from build123d import *

# Parameters (mm, degrees)
FILLET2_R  = 0.1
SKETCH2_W  = 5.5
SKETCH2_H  = 0.8
SLOT_DEPTH = 0.85


with BuildPart() as part:
    # BodySke → Base-Revolve (revolve)
    with BuildSketch(Plane.XY):
        Polygon((2, 1.5), (2, 2.75), (0, 2.575022673), (0, 0), (18, 0), (18, 1.5), align=None)
    revolve(axis=Axis((-25.4, 0, 0), (1, 0, 0)))

    # Fillet2
    fillet2_edges = [part.edges().sort_by_distance(p)[0] for p in [
        (0, -2.575022673, 0),
    ]]
    fillet(fillet2_edges, radius=FILLET2_R)

    # Sketch2 → Slot (cut)
    with BuildSketch(Plane(origin=(0, 0, 0), x_dir=(0, 0, -1), z_dir=(1, 0, 0))):
        Rectangle(SKETCH2_W, SKETCH2_H)
    extrude(amount=SLOT_DEPTH, mode=Mode.SUBTRACT)


solid = part.part
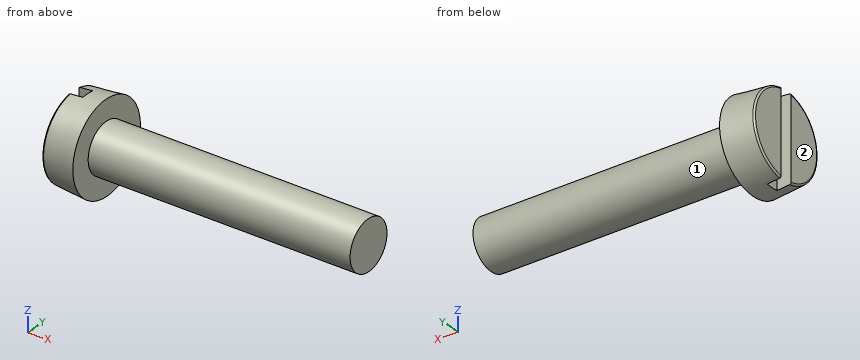
Source: CAD feature listing. Evaluate the final solid. Frame: model axes, mm. Face numbers are marked on the shaded views. A direction names the side the tool comes from. Give positions to 0.01 mm unless a question says otherwise; leave off trailing zeros. Write each loop counter-clockwise with the first axis right and the second up, starting at its lowest first coordinate (ties: lowest second). Pieces come first, ordered by that corner, then holes. Notation, with made-up numbers: M 11.25,42 L 40.25,42 A16 ccw 40.25,58 Z; hole C 50,-10 d1. An arc over 180 degrees is marked long. Return JSON: item names as keys, results as strings. Group by question number.
1) Cut plane A-A, the plane z = 0. Output: boundary loops of the cut face in (x, y).
2) Ray query, L1, parallel to X at y = -1.25, z = 1.5; L2, parallel to Y at x = 4.5, z = 0.1; L3, parallel to Z at x = 2.5, y = -0.8. Return the intervals inside material, ascending.
3) Cut plane C-C, the plane x = 16. Output: boundary loops of the cut face in (y, z).
4) Set-up query: the marked faces 1 and 2. Return all of +Z, -Z, +X, -X, +Y, -Y with unobstructed straight access to the full face (end or side cutting, diameter ignored); none if empty.
5) First-contact query: pin 1 Ø2 at (x, y) = (12, -1) entering from +Z; pin 2 Ø1.5 at (x, y) = (4.5, -1.5) entering from +Z. Flat tips, straight axial feed; report the tip coordinate or a pass-through.
6) Cut plane B-B, the plane y = 0. Output: boundary loops of the cut face in (x, z).
Data:
{
 "1": {"outline": "M 0,-2.48 A0.1 ccw 0.09,-2.58 L 2,-2.75 L 2,-1.5 L 18,-1.5 L 18,1.5 L 2,1.5 L 2,2.75 L 0.09,2.58 A0.1 ccw 0,2.48 L 0,0.4 L 0.85,0.4 L 0.85,-0.4 L 0,-0.4 Z"},
 "2": {"L1": "x = 0 to 2", "L2": "y = -1.5 to 1.5", "L3": "z = -1.27 to 1.27"},
 "3": {"outline": "C 0,0 d3"},
 "4": {"face 1": "+X", "face 2": "+Z, -Z, -X, +Y, -Y"},
 "5": {"pin 1": "stops at z = 1.5", "pin 2": "stops at z = 1.3"},
 "6": {"outline": "M 0.85,-2.65 L 2,-2.75 L 2,-1.5 L 18,-1.5 L 18,1.5 L 2,1.5 L 2,2.75 L 0.85,2.65 Z"}
}
